from build123d import *
from build123d.topology import SkipClean

# Parameters (mm, degrees)
SKETCH_1_R          = 3.5
EXTRUDE_1_DEPTH     = 105
CUT_EXTRUDE_1_DEPTH = 2
SKETCH_3_R          = 3.5
SKETCH_3_R_2        = 2.1
CUT_EXTRUDE_3_DEPTH = 2
SKETCH_4_R          = 0.548210007
EXTRUDE_2_DEPTH     = 2
SKETCH_5_R          = 1.45
CUT_EXTRUDE_5_DEPTH = 10


with BuildPart() as part:
    # 草图1 → 凸台-拉伸1 (new body)
    with BuildSketch(Plane(origin=(0, 0, 0), x_dir=(1, 0, 0), z_dir=(0, 1, 0))):
        with Locations(Location((0, 0, 0), (0, 0, 270))):
            Circle(SKETCH_1_R)
    extrude(amount=EXTRUDE_1_DEPTH)

    # 草图2 → 切除-拉伸1 (cut)
    with BuildSketch(Plane.XZ):
        with BuildLine():
            Line((0, 3.5), (0, 2.1))
            ThreePointArc((0, 2.1), (1.698935688, 1.23434903), (1.997218684, -0.648935688))
            Line((1.997218684, -0.648935688), (3.328697807, -1.08155948))
            ThreePointArc((3.328697807, -1.08155948), (3.456909192, -0.547520628), (3.5, 0))
            ThreePointArc((3.5, 0), (2.474873734, 2.474873734), (0, 3.5))
        make_face()
        with BuildLine():
            ThreePointArc((0, -2.1), (-1.698935688, -1.23434903), (-1.997218684, 0.648935688))
            Line((-1.997218684, 0.648935688), (-3.328697807, 1.08155948))
            ThreePointArc((-3.328697807, 1.08155948), (-2.83155948, -2.057248383), (0, -3.5))
            Line((0, -3.5), (0, -2.1))
        make_face()
    extrude(amount=-CUT_EXTRUDE_1_DEPTH, mode=Mode.SUBTRACT)

    # 草图3 → 切除-拉伸3 (cut)
    with SkipClean():  # the faces are left unmerged after this step: merging them gives an invalid solid
        with BuildSketch(Plane.XZ.offset(-2)):
            with Locations(Location((0, 0, 0), (0, 0, 270))):
                Circle(SKETCH_3_R)
            with Locations(Location((0, 0, 0), (0, 0, 270))):
                Circle(SKETCH_3_R_2, mode=Mode.SUBTRACT)
        extrude(amount=-CUT_EXTRUDE_3_DEPTH, mode=Mode.SUBTRACT)

    # 草图4 → 凸台-拉伸2 (add)
    with BuildSketch(Plane(origin=(0, 2, 0), x_dir=(1, 0, 0), z_dir=(0, 1, 0))):
        with BuildLine():
            ThreePointArc((-1.491392248, -1.478427936), (-1.053967002, -1.816357222), (-0.543519995, -2.028444235))
            ThreePointArc((-0.543519995, -2.028444235), (-0.494470754, -1.90238195), (-0.477782325, -1.768146991))
            ThreePointArc((-0.477782325, -1.768146991), (-0.875331586, -1.241045908), (-1.491392248, -1.478427936))
        make_face()
        with BuildLine():
            ThreePointArc((-1.491392248, -1.478427936), (-1.301132932, -2.242311375), (-0.543519995, -2.028444235))
            ThreePointArc((-0.543519995, -2.028444235), (-1.053967002, -1.816357222), (-1.491392248, -1.478427936))
        make_face()
        with Locations((1.025992333, 1.768146991)):
            Circle(SKETCH_4_R)
    extrude(amount=EXTRUDE_2_DEPTH)

    # 草图5 → 切除-拉伸5 (cut)
    with BuildSketch(Plane(origin=(0, 105, 0), x_dir=(1, 0, 0), z_dir=(0, 1, 0))):
        with Locations(Location((0, 0, 0), (0, 0, 270))):
            Circle(SKETCH_5_R)
    extrude(amount=-CUT_EXTRUDE_5_DEPTH, mode=Mode.SUBTRACT)

    # 草图6 → 切除-旋转2 (revolve, cut)
    with BuildSketch(Plane.XY, mode=Mode.PRIVATE) as cut_revolve_2_sk:
        with BuildLine():
            Line((1.203106705, 105), (1.203106705, 104.958820899))
            add(Edge.make_bspline(
                [(3.5, 104.7), (2.737905529, 104.82566733), (1.972274431, 104.911940963), (1.203106705, 104.958820899)],
                knots=[0, 0, 0, 0, 0.657831992, 0.657831992, 0.657831992, 0.657831992], degree=3))
            Line((3.5, 104.7), (3.5, 105))
            Line((3.5, 105), (1.203106705, 105))
        make_face()
    revolve(cut_revolve_2_sk.sketch.rotate(Axis((0, 107.628853611, 0), (0, -1, 0)), 270), axis=Axis((0, 107.628853611, 0), (0, -1, 0)), mode=Mode.SUBTRACT)


solid = part.part
Source: CAD feature listing. Evaluate the final solid. Frame: model axes, mm. A direction names the side the tool comes from. Give positions to 0.01 mm unless a question says otherwise; leave off trailing zeros. Write each loop counter-clockwise with the first axis right and the second up, starting at its lowest first coordinate (ties: lowest second). Pieces come first, ordered by that corner, then holes. Notation, with made-up numbers: M -1,-18.75 L 14,-18.75 A33 cw 14,12.25 Z; hole C 15,-33 d6. An arc over 180 degrees is marked long. Answer as a JSON object with one key per item and string values.
Q1. Access query for faces 4 (the face through (-2, 4, -2)), 5 (the face through (0, 0, 0)). Directions: +Z, -Z, +X, -X, +Y, -Y. A direction counts if a zero-diameter tool reaches every point of the face in a straight line with its end or side. Return the directions, or none.
Geometry check:
{"face 4": "none", "face 5": "+Z, -Z, +X, -X, -Y"}
Q2. Contact query for flat-ended pins moving along their axis: P1, Ø2.5, axis at x = -2, z = 2, coming from the +Y side; P2, Ø1, axis at y = 51.5, z = 1, coming from the +X side; P3, Ø1.5, axis at y = 0.5, z = 3, coming from the +X side. Output: stop coordinate, or through.
Geometry check:
{"P1": "stops at y = 104.93", "P2": "stops at x = 3.46", "P3": "stops at x = 0"}
Q3. Cut plane A-A, the plane y = 65. Return the cut outline in (x, z), then the cut area to 3 significant figures.
Geometry check:
{"outline": "C 0,0 d7", "area": "38.5 mm^2"}
Q4. Ray query, line 1 along X through (y, z) = (102.25, 0); line 2 along Y through (x, z) = (-2, 2.75); line 3 along Y through (x, z) = (0, 1.5). Return the intervals inside material, ascending.
Geometry check:
{"line 1": "x = -3.5 to -1.45, 1.45 to 3.5", "line 2": "y = 0 to 2, 4 to 104.72", "line 3": "y = 0 to 104.94"}
Q5. Mould query, pull axis Z, two halves, no side actions, for faces 1 (the face through (-2.1, 1, 2.8)), 2 (the face through (0.06, 100.04, -1.45)), 3 (the face through (-3.417, 53.645, -0.759)). Classes: +Z half, -Z half, draft (parallel to the pull), parting line (faces both ways), or undercut.
Geometry check:
{"face 1": "+Z half", "face 2": "undercut", "face 3": "parting line"}
